Part model, mm, in its own coordinate system. A direction names the side the tool comes from. Give positions to 0.01 mm unless a question says otherwise; leave off trailing zeros. Write each loop counter-clockwise with the first axis right and the second up, starting at its lowest first coordinate (ties: lowest second). Pieces come first, ordered by that corner, then holes.
from build123d import *

# Parameters (mm, degrees)
SKETCH1_W           = 40
SKETCH1_H           = 30
BOSS_EXTRUDE1_DEPTH = 3
SKETCH2_R           = 3
CUT_EXTRUDE1_DEPTH  = 1.5
SKETCH3_R           = 1.5
CUT_EXTRUDE2_DEPTH  = 30.193321154
SKETCH4_R           = 5
SKETCH4_R_2         = 3
CUT_EXTRUDE3_DEPTH  = 0.5
SKETCH6_W           = 10
SKETCH6_H           = 1
BOSS_EXTRUDE2_DEPTH = 10
RIB5_REACH          = 42.237
SKETCH10_WALL_W     = 88.876722392
SKETCH10_WALL_H     = 3


with BuildPart() as part:
    # Sketch1 → Boss-Extrude1 (new body)
    with BuildSketch(Plane(origin=(0, 0, 0), x_dir=(1, 0, 0), z_dir=(0, 1, 0))):
        with Locations((-5, 0)):
            Rectangle(SKETCH1_W, SKETCH1_H)
    extrude(amount=BOSS_EXTRUDE1_DEPTH)

    # Sketch2 → Cut-Extrude1 (cut)
    with BuildSketch(Plane(origin=(0, 3, 0), x_dir=(1, 0, 0), z_dir=(0, 1, 0))):
        with Locations(Location((0, 0, 0), (0, 0, 270))):
            Circle(SKETCH2_R)
    extrude(amount=-CUT_EXTRUDE1_DEPTH, mode=Mode.SUBTRACT)

    # Sketch3 → Cut-Extrude2 (cut, through all)
    with BuildSketch(Plane(origin=(0, 1.5, 0), x_dir=(1, 0, 0), z_dir=(0, 1, 0))):
        with Locations(Location((0, 0, 0), (0, 0, 270))):
            Circle(SKETCH3_R)
    extrude(amount=-CUT_EXTRUDE2_DEPTH, mode=Mode.SUBTRACT)

    # Sketch4 → Cut-Extrude3 (cut)
    with BuildSketch(Plane.XZ):
        with Locations(Location((0, 0, 0), (0, 0, 270))):
            Circle(SKETCH4_R)
        with Locations(Location((0, 0, 0), (0, 0, 90))):
            Circle(SKETCH4_R_2, mode=Mode.SUBTRACT)
    extrude(amount=-CUT_EXTRUDE3_DEPTH, mode=Mode.SUBTRACT)

    # Sketch6 → Boss-Extrude2 (add)
    with BuildSketch(Plane(origin=(0, 3, 0), x_dir=(1, 0, 0), z_dir=(0, 1, 0))):
        with Locations((-20, -0.7)):
            Rectangle(SKETCH6_W, SKETCH6_H)
        with Locations((-20, 0.7)):
            Rectangle(SKETCH6_W, SKETCH6_H)
    extrude(amount=BOSS_EXTRUDE2_DEPTH)

    # Sketch10 wall → Rib5 (add, up to next)
    with BuildSketch(Plane(origin=(-20, 5.5, 3.2), x_dir=(0, -0.780868809443, 0.624695047554), z_dir=(0, -0.624695047554, -0.780868809443)), mode=Mode.PRIVATE) as rib5_sk1:
        Rectangle(SKETCH10_WALL_W, SKETCH10_WALL_H)
    rib5_tool1 = extrude(rib5_sk1.sketch, amount=RIB5_REACH, mode=Mode.PRIVATE) - part.part
    rib5 = rib5_tool1.solids().sort_by_distance((-20, 5.5, 3.2))[0]
    add(rib5)

    # Mirror1: Rib5 across plane
    add(rib5.mirror(Plane.XY))


solid = part.part
1) Mould opens along X. For faces 6 (the cylindrical face through (0.45, 0.76, 1.43)), 7 (the flat face through (-25, 2, 0)), 8 (the flat face through (-18.5, 5, 2)) say: +X half, -X half, draft (parallel to the pull), parting line (faces both ways), or undercut.
Check result:
face 6: undercut
face 7: -X half
face 8: +X half
2) Saw through at C-C (y = 4.5). Write the cut outline in (x, z).
Check result:
outline: (-25, -1.2) - (-21.5, -1.2) - (-21.5, -4) - (-18.5, -4) - (-18.5, -1.2) - (-15, -1.2) - (-15, -0.2) - (-25, -0.2) - close; (-25, 0.2) - (-15, 0.2) - (-15, 1.2) - (-18.5, 1.2) - (-18.5, 4) - (-21.5, 4) - (-21.5, 1.2) - (-25, 1.2) - close
3) Saw through at A-A (y = 7.5). Write the cut outline in (x, z).
Check result:
outline: (-25, -1.2) - (-21.5, -1.2) - (-21.5, -1.6) - (-18.5, -1.6) - (-18.5, -1.2) - (-15, -1.2) - (-15, -0.2) - (-25, -0.2) - close; (-25, 0.2) - (-15, 0.2) - (-15, 1.2) - (-18.5, 1.2) - (-18.5, 1.6) - (-21.5, 1.6) - (-21.5, 1.2) - (-25, 1.2) - close
4) Saw through at D-D (x = -13). Write the cut outline in (y, z).
Check result:
outline: (0, -15) - (3, -15) - (3, 15) - (0, 15) - close
5) 3-axis set-ups, long thin cutter, end or side, ignore diameter. For faces 1 (the flat face through (-20, 8, -0.2)), 2 (the flat face through (-15, 8, 1)), 3 (the flat face through (-21.5, 5, 2)), 4 (the flat face through (-20, 9, 1.2)), 5 (the flat face through (-3.3, 0.5, 0.1)): which of +Z, -Z, +X, -X, +Y, -Y reach the whole face in a straight line?
Check result:
face 1: +X, -X, +Y
face 2: +Z, -Z, +X, +Y
face 3: +Z, -X, +Y
face 4: +Z, +Y
face 5: -Y
6) Saw through at B-B (x = 0). Write the cut outline in (y, z), and give its area (3 significant figures).
Check result:
outline: (0, -15) - (3, -15) - (3, -3) - (1.5, -3) - (1.5, -1.5) - (0, -1.5) - (0, -3) - (0.5, -3) - (0.5, -5) - (0, -5) - close; (0, 1.5) - (1.5, 1.5) - (1.5, 3) - (3, 3) - (3, 15) - (0, 15) - (0, 5) - (0.5, 5) - (0.5, 3) - (0, 3) - close
area: 74.5 mm2
7) Flat gauge pins, fed straight in: P1, Ø9.5, axis at x = 0, z = 0, coming from the +Y side; P2, Ø1.1, axis at y = 8.5, z = -0.5, coming from the +X side; P3, Ø3, axis at x = -21, y = 8.5, coming from the +Z side. Where does each tip first touch, or does it go through?
Check result:
P1: stops at y = 3
P2: stops at x = -15
P3: stops at z = 2
8) Drill centre lines: L1, parallel to X at y = 0.25, z = 0; L2, parallel to Z at x = -17, y = 12; L3, parallel to X at y = 0.8, z = 0. Where is each one in solid material? Low to high.
Check result:
L1: x = -25 to -5, -3 to -1.5, 1.5 to 3, 5 to 15
L2: z = -1.2 to -0.2, 0.2 to 1.2
L3: x = -25 to -1.5, 1.5 to 15
